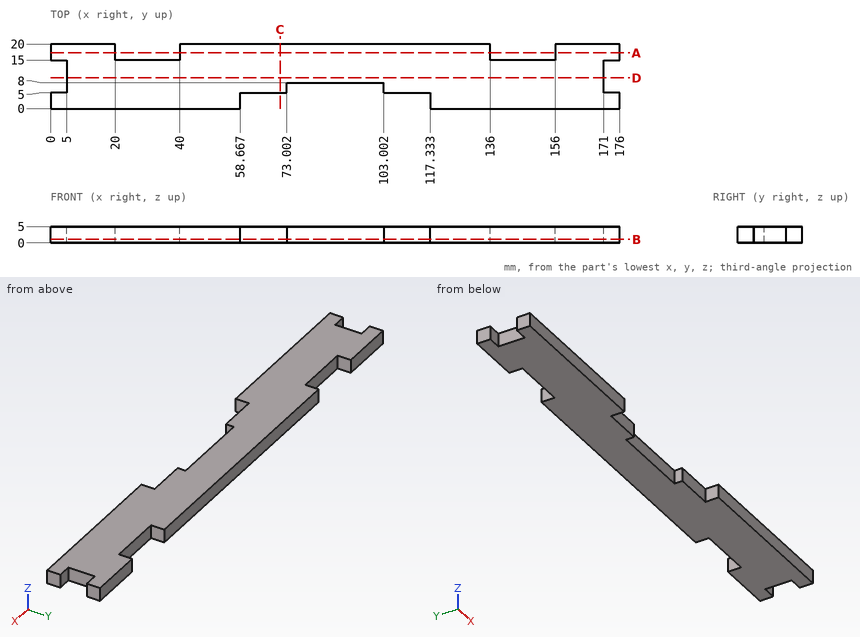
Print and shaded views of the part. All mm, measured from the part's lowest x, y and z. Coordinates: 2 decimals unless noted, no trailing zeros. Order: outer loops, then holes, each group sorted by start corner. A loop starts at its lowest first (then second) coordinate and runs counter-clockwise, first axis right, second up.
(1) Pin check, flat tips, straight feed: pin 1 Ø1.5 at (x, z) = (31, 1.5) entering from +Y; pin 2 Ø1.5 at (x, z) = (63.5, 2) entering from -Y; pin 3 Ø1.5 at (y, z) = (6.5, 1.5) entering from +X. Stop position of each tip, or through.
Check sheet entries:
pin 1: stops at y = 15
pin 2: stops at y = 5
pin 3: stops at x = 171
(2) Slice it at D-D, the plane y = 9.5. Write the cut outline in (x, z), and give its area (3 significant figures).
Check sheet entries:
outline: (5, 0) - (171, 0) - (171, 5) - (5, 5) - close
area: 830 mm2
(3) Slice it at B-B, the plane z = 1.1. Write the cut outline in (x, y), and give its area (3 significant figures).
Check sheet entries:
outline: (0, 0) - (58.67, 0) - (58.67, 5) - (73, 5) - (73, 8) - (103, 8) - (103, 5) - (117.33, 5) - (117.33, 0) - (176, 0) - (176, 5) - (171, 5) - (171, 15) - (176, 15) - (176, 20) - (156, 20) - (156, 15) - (136, 15) - (136, 20) - (40, 20) - (40, 15) - (20, 15) - (20, 20) - (0, 20) - (0, 15) - (5, 15) - (5, 5) - (0, 5) - close
area: 2,840 mm2
(4) Slice it at C-C, the plane x = 71. Write the cut outline in (y, z).
Check sheet entries:
outline: (5, 0) - (20, 0) - (20, 5) - (5, 5) - close
(5) Slice it at A-A, the plane y = 17.25. Write the cut outline in (x, z), and give its area (3 significant figures).
Check sheet entries:
outline: (0, 0) - (20, 0) - (20, 5) - (0, 5) - close; (40, 0) - (136, 0) - (136, 5) - (40, 5) - close; (156, 0) - (176, 0) - (176, 5) - (156, 5) - close
area: 680 mm2
(6) Probe L1, parallel to X at y = 15.5, z = 1.85; L2, parallel to X at y = 4.5, z = 4.35; L3, parallel to Y at x = 32, z = 2.5. List the from-to ranges inside material, lowest first.
Check sheet entries:
L1: x = 0 to 20, 40 to 136, 156 to 176
L2: x = 0 to 58.67, 117.33 to 176
L3: y = 0 to 15
